Could you check a few things on this model? Use its own coordinates, in mm. Give positions to 0.01 mm unless a question says otherwise; leave off trailing zeros. Order: outer loops, then holes, each group sorted by start corner. A loop starts at its lowest first (then second) coordinate and runs counter-clockwise, first axis right, second up. Notation, with made-up numbers: M 30,47.5 L 80,47.5 A20 ccw 80,52.5 Z; hole C -28.5,52 d5. An arc over 180 degrees is marked long. Use a Markdown table: item, result. Add a question column.
Item 1: I'm going to push a flat-ended pin straight in: pin 1 Ø4 at (x, y) = (-9, 22.5) entering from +Z. Where does the tip first touch, or does it pass through?
Item 2: Suppose I cut it at A-A on y = 26. Write out the boundary of the cut face in (x, z).
Item 3: Suppose I cut it at D-D on y = 5. Write out the boundary of the cut face in (x, z), plus the area to 3 significant figures.
Item 4: If I drill on L1, parallel to X at y = 4.5, z = 0.3; L2, parallel to Y at x = 9, z = 0.45; L3, parallel to X at y = 29.5, z = 0.1, over which ranges is the centre line in solid material (lowest first)? Write a range as from..to.
Item 5: Suppose I cut it at C-C on x = -15. Write out the boundary of the cut face in (y, z).
Item 6: Suppose I cut it at B-B on y = 31. Write out the boundary of the cut face in (x, z), plus the area to 3 significant figures.
Item 7: If we mould it in two halves opening along Y, with no side actions, what happens to faces 1 (the face through (2.93, 19.9, 0.25)), 2 (the face through (-21.076, 24.465, 0.246)), 3 (the face through (0, 14, 0))? For each: released by +Y, released by -Y, zero draft, split by the parting line, or undercut.
Autodesk Inventor part; units mm, degrees
ref_plane "Work Plane1" through (-9.001, 17.5, 0) normal (0, 1, 0) x (1, 0, 0)
ref_plane "YZ Plane" through (0, 0, 0) normal (1, 0, 0) x (0, 1, 0)
ref_plane "XZ Plane" through (0, 0, 0) normal (0, 1, 0) x (-1, 0, 0)
sketch "Sketch1" plane through (0, 0, 0) normal (0, 0, 1) x (1, 0, 0)
  line L0 (-32.5, 0) -> (32.5, 0)
  line L1 (32.5, 0) -> (32.5, 13.6)
  line L2 (32.5, 13.6) -> (10, 35)
  line L3 (10, 35) -> (-10, 35)
  line L4 (-10, 35) -> (-32.5, 13.6)
  line L5 (-32.5, 13.6) -> (-32.5, 0)
  line L6 (0, 0) -> (0, 41.5771) construction
  dimension "d0" = 13.6
  dimension "d1" = 65
  dimension "d2" = 35
  dimension "d3" = 20
extrude "Extrusion1" add sketch "Sketch1" along normal blind 0.5
fillet "Fillet1" radius 2.5 4 edges at (-32.5, 13.6, 0.25) (32.5, 13.6, 0.25) (10, 35, 0.25) (-10, 35, 0.25)
sketch "Sketch2" plane through (0, 0, 0.5) normal (0, 0, 1) x (1, 0, 0)
  arc A0 (-9.001, 35) -> (-10.7239, 34.3115) centre (-9.001, 32.5) ccw
  line L0 (9.001, 35) -> (-9.001, 35)
  line L1 (-32.5, 0) -> (32.5, 0)
  point P0 (0, 0)
  point P1 (0, 35)
  point P2 (-30, 12.5)
  point P3 (30, 12.5)
  point P4 (30, 4.5)
  point P5 (-30, 4.5)
  point P6 (0, 0)
  point P7 (-16, 17.5)
  point P8 (16, 17.5)
  point P9 (0, 35)
  dimension "d9" = 60
  dimension "d10" = 30
  dimension "d11" = 4.5
  dimension "d12" = 8
  dimension "d13" = 16
  dimension "d14" = 32
  dimension "d15" = 5
hole "Hole1" at (-16, 17.5, 0.5) at (16, 17.5, 0.5) direction (0, 0, -1) diameter 6 depth 0.5
hole "Hole2" at (-30, 12.5, 0.5) at (30, 12.5, 0.5) at (30, 4.5, 0.5) at (-30, 4.5, 0.5) direction (0, 0, -1) diameter 2.5 depth 0.5
sketch "Sketch3" plane through (0, 0, 0) normal (0, 0, -1) x (-1, 0, 0)
  line L0 (-3.5, 14.5) -> (3.5, 14.5)
  line L1 (3.5, 14.5) -> (3.5, 20.5)
  line L2 (3.5, 20.5) -> (-3.5, 20.5)
  line L3 (-3.5, 20.5) -> (-3.5, 14.5)
  line L4 (-3.5, 14.5) -> (3.5, 20.5) construction
  line L5 (3.5, 14.5) -> (-3.5, 20.5) construction
  circle A0 centre (-16, 17.5) radius 3
  line L6 (32.5, 0) -> (-32.5, 0)
  point P0 (0, 0)
  point P1 (0, 17.5)
  point P2 (-3.5, 17.5)
  point P3 (0, 0)
  dimension "d30" = 7
  dimension "d31" = 6
extrude "Extrusion2" cut sketch "Sketch3" against normal up to surface (0.5 mm away) contours L3 L2 L1 L0
fillet "Fillet2" radius 2 4 edges at (3.5, 20.5, 0.25) (-3.5, 20.5, 0.25) (-3.5, 14.5, 0.25) (3.5, 14.5, 0.25)
sketch "Sketch4" plane through (0, 0, 0) normal (0, 0, -1) x (-1, 0, 0)
  line L0 (-2, 9.5) -> (2, 9.5) construction
  line L1 (-2, 11) -> (2, 11)
  line L2 (2, 8) -> (-2, 8)
  arc A0 (-2, 11) -> (-2, 8) centre (-2, 9.5) ccw
  arc A1 (2, 8) -> (2, 11) centre (2, 9.5) ccw
  line L3 (32.5, 0) -> (-32.5, 0)
  circle A2 centre (30, 12.5) radius 1.25
  point P0 (0, 0)
  point P1 (0, 9.5)
  point P2 (0, 0)
  point P3 (0, 0)
  point P4 (0, 0)
  point P5 (0, 0)
  dimension "d35" = 1.5
  dimension "d37" = 4
  dimension "d39" = 3
  dimension "d40" = 2
extrude "Extrusion3" cut sketch "Sketch4" against normal up to surface (0.5 mm away) contours L1 A1 L2 A0
ref_plane "Work Plane1" through (-9.001, 17.5, 0) normal (0, 1, 0) x (1, 0, 0)
mirror "Mirror1" about plane through (-9.001, 17.5, 0) normal (0, 1, 0) of "Extrusion3"
sketch "Sketch5" plane through (0, 0, 0) normal (0, 0, -1) x (-1, 0, 0)
  circle A0 centre (-30, 12.5) radius 1.25
  line L0 (32.5, 0) -> (-32.5, 0)
  point P0 (0, 0)
  point P1 (-9, 12.5)
  point P2 (9, 12.5)
  point P3 (0, 0)
  point P4 (-9, 4.5)
  point P5 (9, 4.5)
  dimension "d44" = 18
  dimension "d45" = 9
  dimension "d46" = 4.5
hole "Hole3" at (9, 12.5, 0) at (-9, 12.5, 0) at (9, 4.5, 0) at (-9, 4.5, 0) direction (0, 0, 1) diameter 2.5 depth 0.5
mirror "Mirror2" about plane through (-9.001, 17.5, 0) normal (0, 1, 0) of "Hole3"
fillet "Fillet3" radius 2.5 2 edges at (-32.5, 0, 0.25) (32.5, 0, 0.25)
properties part number "16"
Findings below:
| question | item | result |
|---|---|---|
| 1 | pin 1 | stops at z = 0.5 |
| 2 | outline | M -19.46,0 L -3.41,0 L -3.41,0.5 L -19.46,0.5 Z; M 3.41,0 L 19.46,0 L 19.46,0.5 L 3.41,0.5 Z |
| 3 | outline | M -32.5,0 L -31.15,0 L -31.15,0.5 L -32.5,0.5 Z; M -28.85,0 L -10.15,0 L -10.15,0.5 L -28.85,0.5 Z; M -7.85,0 L 7.85,0 L 7.85,0.5 L -7.85,0.5 Z; M 10.15,0 L 28.85,0 L 28.85,0.5 L 10.15,0.5 Z; M 31.15,0 L 32.5,0 L 32.5,0.5 L 31.15,0.5 Z |
| 3 | area | 27.9 mm^2 |
| 4 | L1 | x = -32.5..-31.25, -28.75..-10.25, -7.75..7.75, 10.25..28.75, 31.25..32.5 |
| 4 | L2 | y = 0..3.25, 5.75..11.25, 13.75..21.25, 23.75..29.25, 31.75..35 |
| 4 | L3 | x = -15.78..-9.75, -8.25..8.25, 9.75..15.78 |
| 5 | outline | M 0,0 L 14.67,0 L 14.67,0.5 L 0,0.5 Z; M 20.33,0 L 30.24,0 L 30.24,0.5 L 20.33,0.5 Z |
| 6 | outline | M -14.21,0 L -10.15,0 L -10.15,0.5 L -14.21,0.5 Z; M -7.85,0 L 7.85,0 L 7.85,0.5 L -7.85,0.5 Z; M 10.15,0 L 14.21,0 L 14.21,0.5 L 10.15,0.5 Z |
| 6 | area | 11.9 mm^2 |
| 7 | face 1 | undercut |
| 7 | face 2 | released by +Y |
| 7 | face 3 | zero draft |
